CAD build for the part. Positions are in the model's coordinates, mm. A direction names the side the tool comes from. Give positions to 0.01 mm unless a question says otherwise; leave off trailing zeros. Loops run counter-clockwise (first coordinate to the right, second up) from the corner with the lowest first, then second, coordinate; pieces in that order, holes last. Notation, with made-up numbers: M 57.5,28.25 L 114.5,28.25 A19 ccw 114.5,39.25 Z; hole C -31.75,16 d11. An arc over 180 degrees is marked long. One line per question, with ' | ' between items.
```python
from build123d import *

# Parameters (mm, degrees)
F0_R     = 44.45
F1_DEPTH = 5.08
F2_R     = 5.07999
F4_R     = 28.575
F5_DEPTH = 101.6
F6_D     = 38.1
F6_DEPTH = 38.1
F6_TIP   = 11.4463947925


# Not quite as in the source:
# - a fillet or chamfer is up to 0.001 mm smaller than in the source, because OpenCascade refuses the exact size


with BuildPart() as f1:
    # F0 (on Front) → F1 (new body)
    with BuildSketch(Plane.XZ):
        Circle(F0_R)
    extrude(amount=F1_DEPTH)

    # F2 (radius 5.08 in the source; OpenCascade refuses exactly that, so slightly less here)
    f2_edges = [f1.edges().sort_by_distance(p)[0] for p in [
        (-44.45, 0, 0),
    ]]
    fillet(f2_edges, radius=F2_R)

    # F4 (on face) → F5 (join)
    with BuildSketch(Plane(origin=(0, 0, 0), x_dir=(-1, 0, 0), z_dir=(0, 1, 0))):
        Circle(F4_R)
    extrude(amount=F5_DEPTH)

    # F6
    with Locations(Plane.XZ.offset(5.08)):
        with Locations((0, 0)):
            Hole(F6_D / 2, depth=F6_DEPTH)
            with Locations((0, 0, -(F6_DEPTH + F6_TIP / 2))):  # 118° drill point
                Cone(0, F6_D / 2, F6_TIP, mode=Mode.SUBTRACT)


solid = f1.part
```
Item 1: Mould opens along Z. For faces 1 (the cylindrical face through (28.547, 50.089, 1.256)), 2 (the cylindrical face through (15.12, 14.24, -11.59)), 3 (the flat face through (9, -5.08, -19)) say: pulls with the +Z half, pulls with the -Z half, needs draft (parallel to the pull), parting line crosses it, or undercut.
Conclusion:
face 1: parting line crosses it | face 2: undercut | face 3: needs draft
Item 2: Drop flat-ended pins along their axis: P1, Ø2, axis at y = 79, z = 14, coming from the -X side; P2, Ø2, axis at x = -5, y = 23.5, coming from the -Z side; P3, Ø8, axis at x = -27.5, y = 72.5, coming from the +Z side. Give the stop position or say it passes through.
Conclusion:
P1: x = -25.45 | P2: z = -28.29 | P3: z = 16.26
Item 3: Drill centre lines: line 1 along Z through (x, y) = (0, 23) (3 decimals); line 2 along Z through (x, y) = (-5, 26.5); line 3 along X through (y, z) = (5, 15). Where is each one in solid material? Low to high. Write a range as [from, to].
Conclusion:
line 1: [-28.575, -19.05], [19.05, 28.575] | line 2: [-28.13, -18.38], [18.38, 28.13] | line 3: [-24.32, -11.74], [11.74, 24.32]
Item 4: 3-axis set-ups, long thin cutter, end or side, ignore diameter. For faces 4 (the flat face through (20, 0, 21)), 5 (the conical face through (-2.438, 42.479, 2.236)): which of +Z, -Z, +X, -X, +Y, -Y reach the whole face in a straight line?
Conclusion:
face 4: +Y | face 5: -Y
Item 5: Saw through at B-B on y = 49.5. Give the cut face in (x, z) (3 decimals), and give its area (3 significant figures).
Conclusion:
outline: C 0,0 d57.15 | area: 2,570 mm²
Item 6: Saw through at A-A on y = 28. Give the cut face in (x, z) (3 decimals), and give its area (3 significant figures).
Conclusion:
outline: C 0,0 d57.15; hole C 0,0 d38.1 | area: 1,430 mm²
